```python
from build123d import *

# Parameters (mm, degrees)
F1_DEPTH = 80
F2_R     = 2.6
F3_DEPTH = 25.001
F6_DEPTH = 25
F7_W     = 10
F7_H     = 10
F8_DEPTH = 80.0010001


with BuildPart() as f1:
    # F0 (on Top) → F1 (new body)
    with BuildSketch(Plane.XY):
        with BuildLine():
            Line((0, -16), (0, -25))
            ThreePointArc((0, -25), (25, 0), (0, 25))
            Line((0, 25), (0, 16))
            ThreePointArc((0, 16), (16, 0), (0, -16))
        make_face()
    extrude(amount=F1_DEPTH)

    # F2 (on Right) → F3 (cut, through all)
    with BuildSketch(Plane.YZ):
        with Locations((-20.5, 20)):
            Circle(F2_R)
        with Locations((-20.5, 60)):
            Circle(F2_R)
        with Locations((20.5, 60)):
            Circle(F2_R)
        with Locations((20.5, 20)):
            Circle(F2_R)
    extrude(amount=F3_DEPTH, mode=Mode.SUBTRACT)

    # F5 (on offset) → F6 (cut)
    with BuildSketch(Plane(origin=(6, 0, 0), x_dir=(0, -1, 0), z_dir=(-1, 0, 0))):
        with BuildLine():
            ThreePointArc((15.25, 60), (20.5, 54.75), (25.75, 60))
            ThreePointArc((25.75, 60), (20.5, 65.25), (15.25, 60))
        make_face()
        with BuildLine():
            ThreePointArc((-15.25, 20), (-16.7876893988, 23.7123106012), (-20.5, 25.25))
            ThreePointArc((-20.5, 25.25), (-24.2123106012, 16.2876893988), (-15.25, 20))
        make_face()
    extrude(amount=-F6_DEPTH, mode=Mode.SUBTRACT)

    # F7 (on Top) → F8 (cut, through all)
    with BuildSketch(Plane.XY):
        with Locations((16, 0)):
            Rectangle(F7_W, F7_H)
    extrude(amount=F8_DEPTH, mode=Mode.SUBTRACT)


solid = f1.part
```
Here's how the part is built. I have some questions about the finished solid (model axes, mm). A direction names the side the tool comes from. Coordinates: 2 decimals unless noted, no trailing zeros. Loops run counter-clockwise (first coordinate to the right, second up) from the corner with the lowest first, then second, coordinate; pieces in that order, holes last. Notation, with made-up numbers: (37, -20) -> (84, -20) arc R25 cw to (84, 10) -> close; hole circle Ø5 at (9.5, -14). An arc over 180 degrees is marked (long way). Return JSON: item names as keys, results as strings.
1) If we section it at A-A, the plane x = 2.25: Write out the boundary of the cut face in (y, z), then the cut area to 3 significant figures.
Results below:
{"outline": "(-24.9, 0) -> (-15.84, 0) -> (-15.84, 80) -> (-24.9, 80) -> close; (15.84, 0) -> (24.9, 0) -> (24.9, 80) -> (15.84, 80) -> close; hole circle Ø5.2 at (-20.5, 20); hole circle Ø5.2 at (-20.5, 60); hole circle Ø5.2 at (20.5, 20); hole circle Ø5.2 at (20.5, 60)", "area": "1,360 mm²"}
2) I need wall thicknesses on line 1 (Z direction, x = 5.5, y = 20.5); line 2 (Y direction, x = 6.5, z = 60); line 3 (Y direction, x = 15.25, z = 60). Which ranges of each line are inside material? Lowest first, please. Write a range as from..to.
Results below:
{"line 1": "0..17.4, 22.6..57.4, 62.6..80", "line 2": "-15.25..-14.62, 14.62..17.9, 23.1..24.14", "line 3": "-15.25..-5, 5..17.9"}
3) If we section it at B-B, the plane y = -20.5: Write out the boundary of the cut face in (x, z), then the cut area to 3 significant figures.
Results below:
{"outline": "(0, 0) -> (14.31, 0) -> (14.31, 17.4) -> (0, 17.4) -> close; (0, 22.6) -> (14.31, 22.6) -> (14.31, 54.75) -> (6, 54.75) -> (6, 57.4) -> (0, 57.4) -> close; (0, 62.6) -> (6, 62.6) -> (6, 65.25) -> (14.31, 65.25) -> (14.31, 80) -> (0, 80) -> close", "area": "952 mm²"}
4) If we section it at C-C, the plane z = 10.5: Write out the boundary of the cut face in (x, y).
Results below:
{"outline": "(0, -25) arc R25 ccw to (0, 25) -> (0, 16) arc R16 cw to (15.2, 5) -> (21, 5) -> (21, -5) -> (15.2, -5) arc R16 cw to (0, -16) -> close"}
5) Will these pins go through, and if not, where does the flat tip stop? pin 1 (4 mm diameter, centred on y = -20.5, z = 60, fed in from -X); pin 2 (5 mm diameter, centred on x = 10.5, z = 67.5, fed in from +Y); pin 3 (2.5 mm diameter, centred on y = -22, z = 59, fed in from +X); pin 4 (6 mm diameter, centred on y = 20.5, z = 60, fed in from +X).
Results below:
{"pin 1": "through", "pin 2": "y = 23.69", "pin 3": "x = 6", "pin 4": "x = 17.85"}
6) Thinking about a two-plate mould opening in Y: for faces 4 (the face through (24.994, -0.55, 39.44)), 5 (the face through (9.49, -12.88, 39.44)), 6 (the face through (15, 6, 80)), which applies, +Y half, -Y half, draft (parallel to the pull), parting line (faces both ways), or undercut?
Results below:
{"face 4": "parting line", "face 5": "undercut", "face 6": "draft"}
7) For faces 1 (the face through (18, 5, 39)), 2 (the face through (6.7, 17.9, 60.1)), 3 (the face through (6, -17.7, 60.1)), which set-ups out of +Z, -Z, +X, -X, +Y, -Y let a thin tool reach every point of the face, with its end or its side?
Results below:
{"face 1": "+Z, -Z, -X", "face 2": "+X, -X", "face 3": "+X"}
8) If we section it at D-D, the plane z = 60: Write out the boundary of the cut face in (x, y).
Results below:
{"outline": "(0, -25) arc R25 ccw to (6, -24.27) -> (6, -23.1) -> (0, -23.1) -> close; (0, -17.9) -> (6, -17.9) -> (6, -15.25) -> (19.81, -15.25) arc R25 ccw to (17.45, 17.9) -> (0, 17.9) -> (0, 16) arc R16 cw to (15.2, 5) -> (21, 5) -> (21, -5) -> (15.2, -5) arc R16 cw to (0, -16) -> close; (0, 23.1) -> (9.56, 23.1) arc R25 ccw to (0, 25) -> close"}
